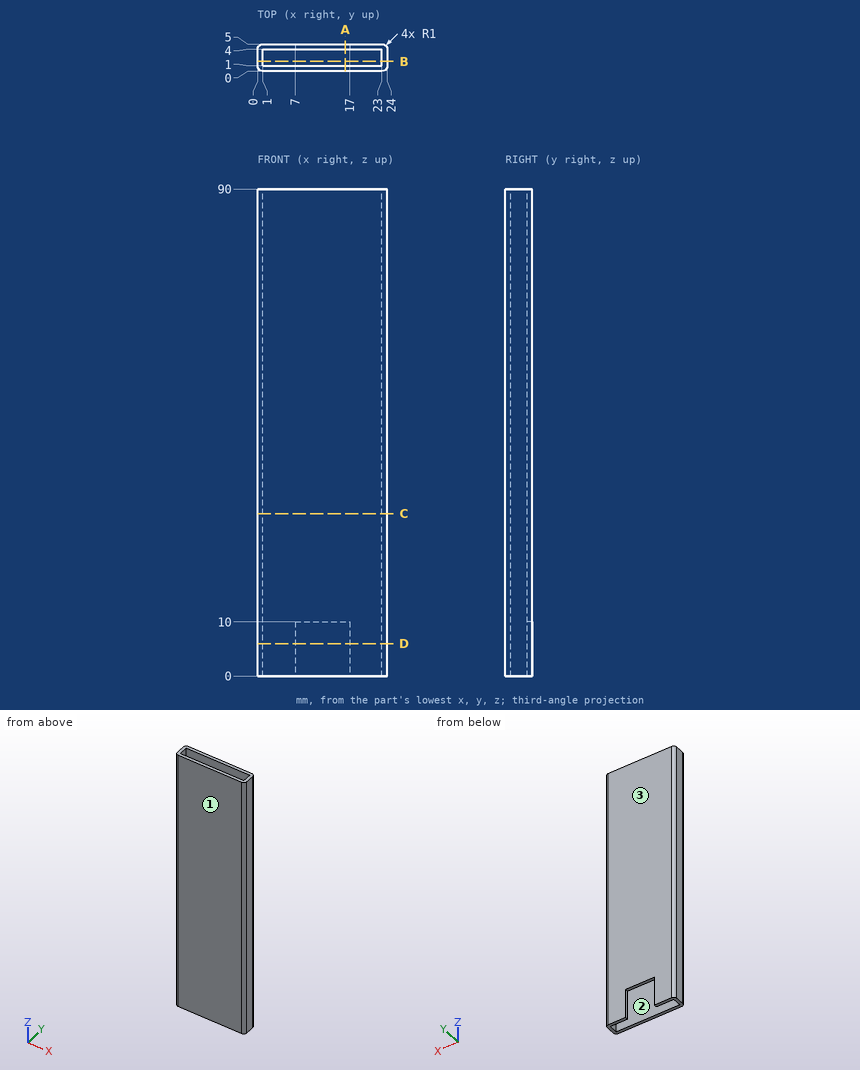
Print and shaded views of the part. All mm, measured from the part's lowest x, y and z. Coordinates: 2 decimals unless noted, no trailing zeros. Order: outer loops, then holes, each group sorted by start corner. A loop starts at its lowest first (then second) coordinate and runs counter-clockwise, first axis right, second up.
(1) Slice it at A-A, the plane x = 16.25. Write the cut outline in (y, z), and give its area (3 significant figures).
Check sheet entries:
outline: (0, 0) - (1, 0) - (1, 90) - (0, 90) - close; (4, 10) - (5, 10) - (5, 90) - (4, 90) - close
area: 170 mm2
(2) Pin check, flat tips, straight feed: pin 1 Ø0.8 at (y, z) = (4.5, 3.5) entering from +X (3 decimals); pin 2 Ø0.5 at (x, y) = (10, 4.5) entering from -Z; pin 3 Ø0.5 at (y, z) = (4.5, 4.5) entering from -X. Stop position of each tip, or through.
Check sheet entries:
pin 1: stops at x = 23.995
pin 2: stops at z = 10
pin 3: stops at x = 0.03
(3) Slice it at C-C, the plane z = 30. Write the cut outline in (x, y).
Check sheet entries:
outline: (0, 1) arc R1 ccw to (1, 0) - (23, 0) arc R1 ccw to (24, 1) - (24, 4) arc R1 ccw to (23, 5) - (1, 5) arc R1 ccw to (0, 4) - close; hole (1, 1) - (23, 1) - (23, 4) - (1, 4) - close
(4) Slice it at D-D, the plane z = 6. Write the cut outline in (x, y), and give its area (3 significant figures).
Check sheet entries:
outline: (0, 1) arc R1 ccw to (1, 0) - (23, 0) arc R1 ccw to (24, 1) - (24, 4) arc R1 ccw to (23, 5) - (17, 5) - (17, 4) - (23, 4) - (23, 1) - (1, 1) - (1, 4) - (7, 4) - (7, 5) - (1, 5) arc R1 ccw to (0, 4) - close
area: 43.1 mm2
(5) Slice it at B-B, the plane y = 1.8. Write the cut outline in (x, z).
Check sheet entries:
outline: (0, 0) - (1, 0) - (1, 90) - (0, 90) - close; (23, 0) - (24, 0) - (24, 90) - (23, 90) - close
(6) Probe L1, parallel to X at y = 1.45, z = 9; L2, parallel to Y at x = 4.5, z = 23; L3, parallel to X at y = 0.75, z = 17. List the from-to ranges inside material, lowest first.
Check sheet entries:
L1: x = 0 to 1, 23 to 24
L2: y = 0 to 1, 4 to 5
L3: x = 0.03 to 23.97
(7) Pull direction Y, two halves, no side cores. Call the marked faces 1, 2 and 3: pulls with the +Y half, pulls with the -Y half, needs draft (parallel to the pull), parting line crosses it, or undercut.
Check sheet entries:
face 1: pulls with the -Y half
face 2: undercut
face 3: pulls with the +Y half
